For this review, take the finished solid that the model builds, in its own axes (mm). Coordinates: 2 decimals unless noted, no trailing zeros. Write each loop counter-clockwise with the first axis right and the second up, starting at its lowest first coordinate (ties: lowest second). Pieces come first, ordered by that corner, then holes. Notation, with made-up numbers: (-28, 79) - (11, 79) arc R18 cw to (11, 110) - close; hole circle Ø10 at (-24.75, 63). An arc over 180 degrees is marked (long way). Use one line per item in the form item = value. Start each with the question number.
1) We need section C-C (y = 6). Give the boundary of the cut face in (x, z).
2) We need section B-B (z = 39.5). Give the boundary of the cut face in (x, y).
3) We need section D-D (x = -4.5). Give the boundary of the cut face in (y, z), plus the area to 3 significant figures.
4) For L1, parallel to Y at x = 0, z = 79; L2, parallel to Y at x = -1.25, z = 10; L3, parallel to X at y = -1.5, z = 8, list the stretches that pass through material, from the lowest coordinate up. Write a range as from..to.
5) Insertion check: P1, Ø2, axis at y = 5, z = 22.5, coming from the -X side; P2, Ø6, axis at x = -3.5, z = 54, coming from the +Y side; P3, Ø4, axis at x = 0, y = 0, coming from the -Z side. Each pin has a flat end and moves straight along its axis. Give the tip position at first contact, or say it passes through.
6) We need section A-A (z = 11). Give the boundary of the cut face in (x, y), plus the area to 3 significant figures.
```python
from build123d import *

# Parameters (mm, degrees)
BOSS_EXTRUDE1_DEPTH         = 88.9
F_1_4_20_TAPPED_HOLE1_D     = 5.1054
F_1_4_20_TAPPED_HOLE1_DEPTH = 16.51
F_1_4_20_TAPPED_HOLE1_TIP   = 1.533816902
F_1_4_20_TAPPED_HOLE2_D     = 5.1054
F_1_4_20_TAPPED_HOLE2_DEPTH = 16.51
F_1_4_20_TAPPED_HOLE2_TIP   = 1.533816902


with BuildPart() as part:
    # Sketch1 → Boss-Extrude1 (new body)
    with BuildSketch(Plane.XY):
        Polygon((6.35, 3.666174209), (0, 7.332348419), (-6.35, 3.666174209), (-6.35, -3.666174209), (0, -7.332348419), (6.35, -3.666174209), align=None)
    extrude(amount=BOSS_EXTRUDE1_DEPTH)

    # 1/4-20 Tapped Hole1
    with Locations(Plane.XY.offset(88.9)):
        with Locations((0, 0)):
            Hole(F_1_4_20_TAPPED_HOLE1_D / 2, depth=F_1_4_20_TAPPED_HOLE1_DEPTH)
            with Locations((0, 0, -(F_1_4_20_TAPPED_HOLE1_DEPTH + F_1_4_20_TAPPED_HOLE1_TIP / 2))):  # 118° drill point
                Cone(0, F_1_4_20_TAPPED_HOLE1_D / 2, F_1_4_20_TAPPED_HOLE1_TIP, mode=Mode.SUBTRACT)

    # 1/4-20 Tapped Hole2
    with Locations(Plane(origin=(0, 0, 0), x_dir=(-1, 0, 0), z_dir=(0, 0, -1))):
        with Locations((0, 0)):
            Hole(F_1_4_20_TAPPED_HOLE2_D / 2, depth=F_1_4_20_TAPPED_HOLE2_DEPTH)
            with Locations((0, 0, -(F_1_4_20_TAPPED_HOLE2_DEPTH + F_1_4_20_TAPPED_HOLE2_TIP / 2))):  # 118° drill point
                Cone(0, F_1_4_20_TAPPED_HOLE2_D / 2, F_1_4_20_TAPPED_HOLE2_TIP, mode=Mode.SUBTRACT)


solid = part.part
```
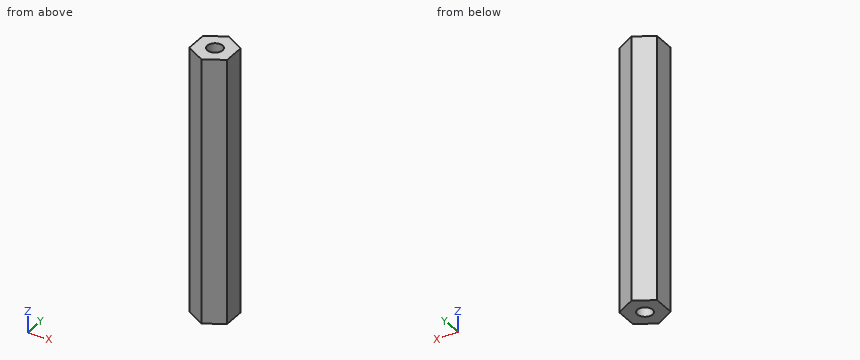
Determined:
q1.outline = (-2.31, 0) - (2.31, 0) - (2.31, 88.9) - (-2.31, 88.9) - close
q2.outline = (-6.35, -3.67) - (0, -7.33) - (6.35, -3.67) - (6.35, 3.67) - (0, 7.33) - (-6.35, 3.67) - close
q3.outline = (-4.73, 0) - (4.73, 0) - (4.73, 88.9) - (-4.73, 88.9) - close
q3.area = 842 mm²
q4.L1 = -7.33..-2.55, 2.55..7.33
q4.L2 = -6.61..-2.23, 2.23..6.61
q4.L3 = -6.35..-2.07, 2.07..6.35
q5.P1 = -5.77
q5.P2 = 7.04
q5.P3 = 16.84
q6.outline = (-6.35, -3.67) - (0, -7.33) - (6.35, -3.67) - (6.35, 3.67) - (0, 7.33) - (-6.35, 3.67) - close; hole circle Ø5.11 at (0, 0)
q6.area = 119 mm²
